Can you work these out from the model? Positions are in its coordinate system, mm. A direction names the side the tool comes from. Coordinates: 2 decimals unless noted, no trailing zeros. Order: outer loops, then holes, each group sorted by start corner. A loop starts at its lowest first (then second) coordinate and runs counter-clockwise, first axis right, second up. Notation, with made-up numbers: (-28, 52) -> (9, 52) arc R33 ccw to (9, 89) -> close; hole circle Ø5 at (-14.5, 7.25). An arc over 180 degrees is marked (long way). Return JSON: item names as keys, results as strings. Group by question number.
1) If I drill on probe 1 along Z at (x, y) = (-0.5, -3); probe 2 along Y at (x, z) = (-0.75, -1); probe 3 along X at (y, z) = (2, -100), over which ranges is the centre line in solid material (lowest first)? Write a range as from..to.
2) If we section it at B-B, the plane z = -6: Please give me the cut outline in (x, y), then the cut area to 3 significant figures.
3) If we section it at A-A, the plane y = 0: Please give me the cut outline in (x, z), then the cut area to 3 significant figures.
4) For pin 1 (10 mm diameter, centred on x = -6, z = -58.5, fed in from -Y); pin 2 (8 mm diameter, centred on x = 4, z = -6, fed in from -Y); pin 3 (1 mm diameter, centred on y = 0.5, z = -60, fed in from +X), each with a flat end and sliding along its axis, tell me the tip position at first contact or that it passes through.
5) If we section it at C-C, the plane z = -85: Please give me the cut outline in (x, y) (3 decimals), then the cut area to 3 significant figures.
6) Thinking about a two-plate mould opening in Y: for faces 1 (the flat face through (0, 0, 6.5)), 2 (the flat face through (6.5, 0, 5)), 3 (the cylindrical face through (3.695, -1.532, -39.694)), 4 (the flat face through (-3.2, -5.66, 4.94)), which applies, +Y half, -Y half, draft (parallel to the pull), parting line (faces both ways), or undercut?
7) For faces 5 (the flat face through (-3.3, 5.6, 4.9)), 6 (the flat face through (0, 0, -110)), 7 (the flat face through (3.3, -5.6, 4.9)), 8 (the cylindrical face through (3.504, -1.823, -95.21)), 9 (the flat face through (3.2, 5.66, 4.94)), which set-ups out of +Z, -Z, +X, -X, +Y, -Y let a thin tool reach every point of the face, with its end or its side?
from build123d import *

# Parameters (mm, degrees)
HEAD_DEPTH     = 8
SHANK_SKETCH_R = 4
SHANK_DEPTH    = 110
SKETCH6_R      = 5.6875
HEAD_CUT_DEPTH = 1.5
FILLET1_R      = 2
FILLET2_R      = 0.5
THREAD_END_W   = 30
THREAD_END_H   = 0.05


with BuildPart() as part:
    # Head Sketch → Head (new body)
    with BuildSketch(Plane.XY):
        Polygon((0, 7.505553499), (6.5, 3.75277675), (6.5, -3.75277675), (0, -7.505553499), (-6.5, -3.75277675), (-6.5, 3.75277675), align=None)
    extrude(amount=HEAD_DEPTH)

    # Shank Sketch → Shank (add)
    with BuildSketch(Plane.XY):
        Circle(SHANK_SKETCH_R)
    extrude(amount=-SHANK_DEPTH)

    # Sketch3 → Flange (revolve)
    with BuildSketch(Plane(origin=(0, 0, 0), x_dir=(-1, 0, 0), z_dir=(0, 1, 0)), mode=Mode.PRIVATE) as flange_sk:
        with BuildLine():
            Line((-8.5, 0), (0, 0))
            Line((0, 0), (0, 5))
            ThreePointArc((0, 5), (-4.909972075, 3.90244066), (-8.885269122, 0.818696884))
            ThreePointArc((-8.885269122, 0.818696884), (-8.952409351, 0.287101482), (-8.5, 0))
        make_face()
    revolve(flange_sk.sketch.rotate(Axis((0, 0, 0), (0, 0, 1)), 30), axis=Axis((0, 0, 0), (0, 0, 1)))

    # Sketch5 → Head Trim (revolve, cut)
    with BuildSketch(Plane(origin=(0, 0, 0), x_dir=(0, 0, -1), z_dir=(1, 0, 0)), mode=Mode.PRIVATE) as head_trim_sk:
        with BuildLine():
            Line((-8, -5.505553499), (-8, -7.505553499))
            Line((-8, -7.505553499), (-6, -7.505553499))
            ThreePointArc((-6, -7.505553499), (-7.414213562, -6.919767062), (-8, -5.505553499))
        make_face()
    revolve(head_trim_sk.sketch.rotate(Axis((0, 0, 15.085599173), (0, 0, -1)), 90), axis=Axis((0, 0, 15.085599173), (0, 0, -1)), mode=Mode.SUBTRACT)

    # Sketch6 → Head Cut (cut)
    with BuildSketch(Plane.XY.offset(8)):
        Circle(SKETCH6_R)
    extrude(amount=-HEAD_CUT_DEPTH, mode=Mode.SUBTRACT)

    # Fillet1
    # the kernel refuses this fillet: 2 mm, written as the material it adds along each edge
    with BuildSketch(Plane(origin=(0, 0, 6.5), x_dir=(1, 0, 0), z_dir=(0, -1, 0))) as fillet1_piece_1:
        with BuildLine():
            CenterArc((3.753168618, 2), FILLET1_R, 270, 75.276973149)
            Line((3.753168618, 0), (3.753168618, -0.04))
            Line((3.753168618, -0.04), (5.6875, -0.04))
            Line((5.6875, -0.04), (5.7275, 0))
            ThreePointArc((5.7275, 0), (5.7275, 0.745853336), (5.726186628, 1.481540806))
            Line((5.726186628, 1.481540806), (5.6875, 1.491706673))
        make_face()
    revolve(axis=Axis((0, 0, 6.5), (0, 0, 1)), revolution_arc=180.000000894)
    with BuildSketch(Plane(origin=(0, 0, 6.5), x_dir=(-0.9999999999999999, -1.560445893577358e-08, 0), z_dir=(-1.560445893577358e-08, 0.9999999999999999, 0))) as fillet1_piece_2:
        with BuildLine():
            CenterArc((3.753168618, 2), FILLET1_R, 270, 75.276973149)
            Line((3.753168618, 0), (3.753168618, -0.04))
            Line((3.753168618, -0.04), (5.6875, -0.04))
            Line((5.6875, -0.04), (5.7275, 0))
            ThreePointArc((5.7275, 0), (5.7275, 0.745853336), (5.726186628, 1.481540806))
            Line((5.726186628, 1.481540806), (5.6875, 1.491706673))
        make_face()
    revolve(axis=Axis((0, 0, 6.5), (0, 0, 1)), revolution_arc=179.999999106)

    # Fillet2
    fillet2_edges = [part.edges().sort_by_distance(p)[0] for p in [
        (-4, 0, 0),
    ]]
    fillet(fillet2_edges, radius=FILLET2_R)

    # Thread End → Thread Cut (revolve, cut)
    with BuildSketch(Plane(origin=(0, 0, 0), x_dir=(0, 0, -1), z_dir=(1, 0, 0)), mode=Mode.PRIVATE) as thread_cut_sk:
        with Locations((95, 3.975)):
            Rectangle(THREAD_END_W, THREAD_END_H)
    revolve(thread_cut_sk.sketch.rotate(Axis((0, 0, -21.551935625), (0, 0, -1)), 60.000022404), axis=Axis((0, 0, -21.551935625), (0, 0, -1)), mode=Mode.SUBTRACT)


solid = part.part
Result sheet:
{
 "1": {"probe 1": "z = -110..6.5", "probe 2": "y = -3.93..3.93", "probe 3": "x = -3.41..3.41"},
 "2": {"outline": "circle Ø8 at (0, 0)", "area": "50.3 mm2"},
 "3": {"outline": "(-8.89, 0.82) arc R0.5 ccw to (-8.5, 0) -> (-4.5, 0) arc R0.5 cw to (-4, -0.5) -> (-4, -80) -> (-3.95, -80) -> (-3.95, -110) -> (3.95, -110) -> (3.95, -80) -> (4, -80) -> (4, -0.5) arc R0.5 cw to (4.5, 0) -> (8.5, 0) arc R0.5 ccw to (8.89, 0.82) arc R11.53 ccw to (6.5, 2.99) -> (6.5, 7.74) arc R2 ccw to (5.69, 7.99) arc R2 cw to (3.75, 6.5) -> (-3.75, 6.5) arc R2 cw to (-5.69, 7.99) arc R2 ccw to (-6.5, 7.74) -> (-6.5, 2.99) arc R11.53 ccw to start", "area": "975 mm2"},
 "4": {"pin 1": "stops at y = -3.87", "pin 2": "stops at y = -4", "pin 3": "stops at x = 4"},
 "5": {"outline": "circle Ø7.9 at (0, 0)", "area": "49.0 mm2"},
 "6": {"face 1": "undercut", "face 2": "draft", "face 3": "parting line", "face 4": "-Y half"},
 "7": {"face 5": "+Z, -X, +Y", "face 6": "-Z, +X, -X, +Y, -Y", "face 7": "+Z, +X, -Y", "face 8": "-Z", "face 9": "+Z, +X, +Y"}
}
